```python
from build123d import *

# Parameters (mm, degrees)
F0_W     = 130
F0_H     = 40
F0_R     = 1.5
F0_R_2   = 15.1
F1_DEPTH = 8
F3_DEPTH = 8
F4_R     = 2.25
F5_DEPTH = 8.001
F6_R     = 5


with BuildPart() as f1:
    # F0 (on Top) → F1 (new body)
    with BuildSketch(Plane.XY):
        Rectangle(F0_W, F0_H)
        with Locations((-61.263456, -16.263456)):
            Circle(F0_R, mode=Mode.SUBTRACT)
        with Locations((-28.736544, -16.263456)):
            Circle(F0_R, mode=Mode.SUBTRACT)
        with Locations((-45, 0)):
            Circle(F0_R_2, mode=Mode.SUBTRACT)
        with Locations((-61.263456, 16.263456)):
            Circle(F0_R, mode=Mode.SUBTRACT)
        with Locations((-28.736544, 16.263456)):
            Circle(F0_R, mode=Mode.SUBTRACT)
    extrude(amount=F1_DEPTH)

    # F2 (on face) → F3 (join)
    with BuildSketch(Plane.XY.offset(8)):
        Polygon((65, 20), (65, 114), (45, 114), (-65, 20), align=None)
    extrude(amount=-F3_DEPTH)

    # F4 (on face) → F5 (cut, through all)
    with BuildSketch(Plane.XY.offset(8)):
        Polygon((-15, 36.419495), (-15, 0), (45, 0), (45, 87.692222), align=None)
        with Locations((55, 99.770185)):
            Circle(F4_R)
        with Locations((55, 47)):
            Circle(F4_R)
        with Locations((55, -11.382008)):
            Circle(F4_R)
    extrude(amount=-F5_DEPTH, mode=Mode.SUBTRACT)

    # F6
    f6_edges = [f1.edges().sort_by_distance(p)[0] for p in [
        (45, 114, 4),
        (-15, 36.419495, 4),
        (45, 87.692222, 4),
        (45, 0, 4),
        (-15, 0, 4),
    ]]
    fillet(f6_edges, radius=F6_R)


solid = f1.part
```
Check sheet for the modelled part. Datum: model origin and axes. Units: mm. A direction names the side the tool comes from. Coordinates: 2 decimals unless noted, no trailing zeros. Write each loop counter-clockwise with the first axis right and the second up, starting at its lowest first coordinate (ties: lowest second). Pieces come first, ordered by that corner, then holes. Notation, with made-up numbers: (38, 24) -> (63, 24) arc R20 ccw to (63, 35) -> close; hole circle Ø9 at (80.5, 59.25). An arc over 180 degrees is marked (long way). Use a Markdown table: item, result.
1. Sectioned sample at A-A (x = 55). Enter the section's corners in (y, z), plus the area to 3 significant figures.
Reported:
| item | result |
|---|---|
| outline | (-20, 0) -> (-13.63, 0) -> (-13.63, 8) -> (-20, 8) -> close; (-9.13, 0) -> (44.75, 0) -> (44.75, 8) -> (-9.13, 8) -> close; (49.25, 0) -> (97.52, 0) -> (97.52, 8) -> (49.25, 8) -> close; (102.02, 0) -> (114, 0) -> (114, 8) -> (102.02, 8) -> close |
| area | 964 mm2 |
2. Sectioned sample at D-D (x = -47). Enter the section's corners in (y, z).
Reported:
| item | result |
|---|---|
| outline | (-20, 0) -> (-14.97, 0) -> (-14.97, 8) -> (-20, 8) -> close; (14.97, 0) -> (35.38, 0) -> (35.38, 8) -> (14.97, 8) -> close |
3. Scan lines: line 1 along Y through (x, z) = (55, 3); line 2 along Y through (x, z) = (-28, 5.75); line 3 along X through (y, z) = (48, 0.75). Record each from-to range of solid material in increasing order.
Reported:
| item | result |
|---|---|
| line 1 | y = -20 to -13.63, -9.13 to 44.75, 49.25 to 97.52, 102.02 to 114 |
| line 2 | y = -20 to -17.57, -14.96 to 14.96, 17.57 to 51.62 |
| line 3 | x = -32.23 to -1.45, 45 to 52.98, 57.02 to 65 |
4. Sectioned sample at C-C (z = 1.25). Give the number of separate pieces and of enclosed holes in the cut face, plus the area to 3 significant figures.
Reported:
| item | result |
|---|---|
| separate pieces | 1 |
| enclosed holes | 9 |
| area | 7,770 mm2 |
5. Release check for a two-part mould opening along X. For faces 3 (the cylindrical face through (45.14, 113.7, 3.94)), 4 (the cylindrical face through (-62.369, 17.277, 3.944)), 5 (the flat face through (-1, -20, 4)) record: pulls with the +X half, pulls with the -X half, needs draft (parallel to the pull), parting line crosses it, or undercut.
Reported:
| item | result |
|---|---|
| face 3 | pulls with the -X half |
| face 4 | undercut |
| face 5 | needs draft |
6. Sectioned sample at B-B (y = 61.5). Enter the section's corners in (x, z).
Reported:
| item | result |
|---|---|
| outline | (-16.44, 0) -> (14.35, 0) -> (14.35, 8) -> (-16.44, 8) -> close; (45, 0) -> (65, 0) -> (65, 8) -> (45, 8) -> close |
7. Tool access check on faces 1 (the flat face through (56, 114, 4)), 2 (the cylindrical face through (42.16, 81.35, 3.94)). Record the directions out of +Z, -Z, +X, -X, +Y, -Y that give a thin tool (end or side, any length) a straight path to the whole face; none if there is none.
Reported:
| item | result |
|---|---|
| face 1 | +Z, -Z, +X, -X, +Y |
| face 2 | +Z, -Z |
8. Go/stop test with flat-tipped pins: pin 1 Ø2 at (x, z) = (-17, 2.5) entering from +Y; pin 2 Ø2.5 at (x, y) = (55, -11.38) entering from +Z. Record where each tip stops, or that it passes through.
Reported:
| item | result |
|---|---|
| pin 1 | stops at y = 61.87 |
| pin 2 | passes through |
